from build123d import *

# Parameters (mm, degrees)
EXTRUDE_1_DEPTH     = 150
CUT_EXTRUDE_2_REACH = 302
SKETCH_3_W          = 7
SKETCH_3_H          = 1.5
CUT_EXTRUDE_START   = -5
SKETCH_4_R          = 2.25
CUT_EXTRUDE_3_DEPTH = 5
SKETCH_5_R          = 3.9
CUT_EXTRUDE_4_DEPTH = 2.5


with BuildPart() as part:
    # 草图1 → 凸台-拉伸1 (new body, symmetric)
    with BuildSketch(Plane.XY):
        Polygon((7.5, 9), (7.5, 6.5), (5, 6.5), (5, 8.5), (3, 8.5), (3, 5), (0, 5), (0, 3.5), (2, 3.5), (2, 1.5), (0, 1.5), (0, 0), (30, 0), (30, 1.5), (28, 1.5), (28, 3.5), (30, 3.5), (30, 5), (27, 5), (27, 8.5), (25, 8.5), (25, 6.5), (22.5, 6.5), (22.5, 9), (19, 9), (19, 7), (21, 5), (9, 5), (11, 7), (11, 9), align=None)
    extrude(amount=EXTRUDE_1_DEPTH, both=True)

    # 草图3 → 切除-拉伸2 (cut, up to next)
    with BuildSketch(Plane.XY.offset(150), mode=Mode.PRIVATE) as cut_extrude_2_sk1:
        with Locations((8.5, 0.75)):
            Rectangle(SKETCH_3_W, SKETCH_3_H)
    cut_extrude_2_tool1 = extrude(cut_extrude_2_sk1.sketch, amount=-CUT_EXTRUDE_2_REACH, mode=Mode.PRIVATE) & part.part
    add(cut_extrude_2_tool1.solids().sort_by_distance((8.5, 0.75, 150))[0], mode=Mode.SUBTRACT)
    # 草图3 → 切除-拉伸2 (cut, up to next)
    with BuildSketch(Plane.XY.offset(150), mode=Mode.PRIVATE) as cut_extrude_2_sk2:
        with Locations((21.5, 0.75)):
            Rectangle(SKETCH_3_W, SKETCH_3_H)
    cut_extrude_2_tool2 = extrude(cut_extrude_2_sk2.sketch, amount=-CUT_EXTRUDE_2_REACH, mode=Mode.PRIVATE) & part.part
    add(cut_extrude_2_tool2.solids().sort_by_distance((21.5, 0.75, 150))[0], mode=Mode.SUBTRACT)
    # 草图3 → 切除-拉伸2 (cut, up to next)
    with BuildSketch(Plane.XY.offset(150), mode=Mode.PRIVATE) as cut_extrude_2_sk3:
        Polygon((14.133974596, 5), (15.866025404, 5), (15, 4.5), align=None)
    cut_extrude_2_tool3 = extrude(cut_extrude_2_sk3.sketch, amount=-CUT_EXTRUDE_2_REACH, mode=Mode.PRIVATE) & part.part
    add(cut_extrude_2_tool3.solids().sort_by_distance((15, 4.833333, 150))[0], mode=Mode.SUBTRACT)

    # 草图4 → 切除-拉伸3 (cut)
    with BuildSketch(Plane(origin=(0, 5, 0), x_dir=(1, 0, 0), z_dir=(0, 1, 0)).offset(CUT_EXTRUDE_START)):
        with Locations(Location((15, 142.5, 0), (0, 0, 90))):  # turned: the seam where the file's is
            Circle(SKETCH_4_R)
    cut_extrude_3 = extrude(amount=CUT_EXTRUDE_3_DEPTH, mode=Mode.SUBTRACT)

    # 草图5 → 切除-拉伸4 (cut)
    with BuildSketch(Plane(origin=(0, 5, 0), x_dir=(1, 0, 0), z_dir=(0, 1, 0))):
        with Locations(Location((15, 142.5, 0), (0, 0, 270))):  # turned: the seam where the file's is
            Circle(SKETCH_5_R)
    cut_extrude_4 = extrude(amount=-CUT_EXTRUDE_4_DEPTH, mode=Mode.SUBTRACT)

    # 镜向1: 切除-拉伸3, 切除-拉伸4 across plane
    add(cut_extrude_3.mirror(Plane.XY), mode=Mode.SUBTRACT)
    add(cut_extrude_4.mirror(Plane.XY), mode=Mode.SUBTRACT)


solid = part.part
Design review of the part built by this model. Coordinates are the model's own, in mm. A direction names the side the tool comes from. Coordinates: 2 decimals unless noted, no trailing zeros. Use one line per item in the form item = value. Start each with the question number.
(1) Insertion check: pin 1 (2 mm diameter, centred on y = 7.5, z = -24, fed in from -X); pin 2 (2 mm diameter, centred on y = 7.5, z = -22, fed in from +X); pin 3 (0.8 mm diameter, centred on x = 6.5, z = 47, fed in from +Y). Each pin has a flat end and moves straight along its axis. Give the tip position at first contact, or say it passes through.
(2) For probe 1 along Z at (x, y) = (15, 4.4); probe 2 along X at (y, z) = (0.7, -142.5); probe 3 along X at (y, z) = (7.5, -127), list the stretches that pass through material, from the lowest coordinate up.
(3) The part is to be moulded in two halves that separate along X. For faces 4 (the flat face through (15, 4, -150)), 5 (the flat face through (8, 1.5, 2)), 6 (the flat face through (13, 2.5, -141)), say which applies: +X half, -X half, draft (parallel to the pull), parting line (faces both ways), or undercut.
(4) For faces 1 (the flat face through (21, 1.5, 2)), 2 (the flat face through (13, 2.5, 141)), 3 (the flat face through (15, 4, 150)), list the 3-axis set-ups (+Z, -Z, +X, -X, +Y, -Y) from which the entire face can be reached by the end or side of a thin tool; tool diameter is ignored.
Answer block:
q1.pin_1 = 3
q1.pin_2 = 27
q1.pin_3 = 6.5
q2.probe_1 = -150 to -146.4, -138.6 to 138.6, 146.4 to 150
q2.probe_2 = 0 to 5, 12 to 12.75, 17.25 to 18, 25 to 30
q2.probe_3 = 3 to 5, 7.5 to 11, 19 to 22.5, 25 to 27
q3.face_4 = draft
q3.face_5 = undercut
q3.face_6 = undercut
q4.face_1 = +Z, -Z, -Y
q4.face_2 = +Y
q4.face_3 = +Z, +X, -X, +Y, -Y
